from build123d import *

# Parameters (mm, degrees)
CROQUIS1_W              = 44
CROQUIS1_H              = 31
CROQUIS1_R              = 1
CROQUIS1_R_2            = 2.1
SALIENTE_EXTRUIR1_DEPTH = 6
CROQUIS2_W              = 31
CROQUIS2_H              = 6
SALIENTE_EXTRUIR2_DEPTH = 16.5
CROQUIS3_R              = 1.1
CROQUIS3_W              = 20.5
CROQUIS3_H              = 41
SALIENTE_EXTRUIR3_DEPTH = 6
CROQUIS4_R              = 2.1
CROQUIS4_R_2            = 1
SALIENTE_EXTRUIR4_DEPTH = 2
CROQUIS5_R              = 2.1
CORTAR_EXTRUIR1_DEPTH   = 3.5
REDONDEO1_R             = 15.5
CHAFL_N1_SIZE           = 2
CHAFL_N2_SIZE           = 2
CHAFL_N3_SIZE           = 4
CHAFL_N4_SIZE           = 4
CHAFL_N5_SIZE           = 7.5


with BuildPart() as part:
    # Croquis1 → Saliente-Extruir1 (new body)
    with BuildSketch(Plane(origin=(0, 0, 0), x_dir=(1, 0, 0), z_dir=(0, 1, 0))):
        Rectangle(CROQUIS1_W, CROQUIS1_H)
        with Locations(Location((13, 0, 0), (0, 0, 270))):
            Circle(CROQUIS1_R, mode=Mode.SUBTRACT)
        with Locations(Location((0, 0, 0), (0, 0, 270))):
            Circle(CROQUIS1_R_2, mode=Mode.SUBTRACT)
        with Locations(Location((7, 0, 0), (0, 0, 270))):
            Circle(CROQUIS1_R, mode=Mode.SUBTRACT)
        with Locations(Location((-7, 0, 0), (0, 0, 270))):
            Circle(CROQUIS1_R, mode=Mode.SUBTRACT)
        with Locations(Location((-10, 0, 0), (0, 0, 270))):
            Circle(CROQUIS1_R, mode=Mode.SUBTRACT)
        with Locations(Location((-13, 0, 0), (0, 0, 270))):
            Circle(CROQUIS1_R, mode=Mode.SUBTRACT)
        with Locations(Location((-16, 0, 0), (0, 0, 270))):
            Circle(CROQUIS1_R, mode=Mode.SUBTRACT)
        with Locations(Location((10, 0, 0), (0, 0, 270))):
            Circle(CROQUIS1_R, mode=Mode.SUBTRACT)
        with Locations(Location((16, 0, 0), (0, 0, 270))):
            Circle(CROQUIS1_R, mode=Mode.SUBTRACT)
    extrude(amount=SALIENTE_EXTRUIR1_DEPTH)

    # Croquis2 → Saliente-Extruir2 (add)
    with BuildSketch(Plane(origin=(22, 0, 0), x_dir=(0, 0, -1), z_dir=(1, 0, 0))):
        with Locations((0, 3)):
            Rectangle(CROQUIS2_W, CROQUIS2_H)
    extrude(amount=SALIENTE_EXTRUIR2_DEPTH)

    # Croquis3 → Saliente-Extruir3 (add)
    with BuildSketch(Plane(origin=(38.5, 0, 0), x_dir=(0, 0, -1), z_dir=(1, 0, 0))):
        Polygon((15.5, 105), (-14.991801075, 105), (-14.991801075, 6), (-15.5, 6), (-15.5, 0), (15.5, 0), align=None)
        with Locations((-4.741801075, 53.5)):
            Circle(CROQUIS3_R, mode=Mode.SUBTRACT)
        with Locations((-4.741801075, 101.5)):
            Circle(CROQUIS3_R, mode=Mode.SUBTRACT)
        with Locations((5.258198925, 53.5)):
            Circle(CROQUIS3_R, mode=Mode.SUBTRACT)
        with Locations((0.258198925, 77.5)):
            Rectangle(CROQUIS3_W, CROQUIS3_H, mode=Mode.SUBTRACT)
        with Locations((5.258198925, 101.5)):
            Circle(CROQUIS3_R, mode=Mode.SUBTRACT)
    extrude(amount=SALIENTE_EXTRUIR3_DEPTH)

    # Croquis4 → Saliente-Extruir4 (add)
    with BuildSketch(Plane.XZ):
        with Locations(Location((0, 0, 0), (0, 0, 270))):
            Circle(CROQUIS4_R)
        with Locations(Location((0, 0, 0), (0, 0, 270))):
            Circle(CROQUIS4_R_2, mode=Mode.SUBTRACT)
    extrude(amount=-SALIENTE_EXTRUIR4_DEPTH)

    # Croquis5 → Cortar-Extruir1 (cut)
    with BuildSketch(Plane(origin=(0, 6, 0), x_dir=(1, 0, 0), z_dir=(0, 1, 0))):
        with Locations((-13, 0)):
            Circle(CROQUIS5_R)
        with Locations((13, 0)):
            Circle(CROQUIS5_R)
    extrude(amount=-CORTAR_EXTRUIR1_DEPTH, mode=Mode.SUBTRACT)

    # Redondeo1
    redondeo1_edges = [part.edges().sort_by_distance(p)[0] for p in [
        (-22, 3, 15.5),
        (-22, 3, -15.5),
    ]]
    fillet(redondeo1_edges, radius=REDONDEO1_R - 0.0001)  # a hair under: the kernel refuses the full size

    # Chaflán1
    chafl_n1_edges = [part.edges().sort_by_distance(p)[0] for p in [
        (18.99995, 0, 15.5),
        (18.99995, 0, -15.5),
        (-17.460184398, 0, -10.960184398),
        (-17.460184398, 0, 10.960184398),
        (44.5, 52.5, -15.5),
        (44.5, 55.5, 14.991801075),
    ]]
    chamfer(chafl_n1_edges, length=CHAFL_N1_SIZE)

    # Chaflán2
    chafl_n2_edges = [part.edges().sort_by_distance(p)[0] for p in [
        (44.5, 4, 15.5),
    ]]
    chamfer(chafl_n2_edges, length=CHAFL_N2_SIZE)

    # Chaflán3
    chafl_n3_edges = [part.edges().sort_by_distance(p)[0] for p in [
        (44.5, 0, 0),
    ]]
    chamfer(chafl_n3_edges, length=CHAFL_N3_SIZE - 0.0001)  # a hair under: the kernel refuses the full size

    # Chaflán4
    chafl_n4_edges = [part.edges().sort_by_distance(p)[0] for p in [
        (38.5, 6, -0.254099463),
    ]]
    chamfer(chafl_n4_edges, length=CHAFL_N4_SIZE)

    # Chaflán5
    chafl_n5_edges = [part.edges().sort_by_distance(p)[0] for p in [
        (40.5, 105, 14.991801075),
        (40.5, 105, -15.5),
    ]]
    chamfer(chafl_n5_edges, length=CHAFL_N5_SIZE)


solid = part.part
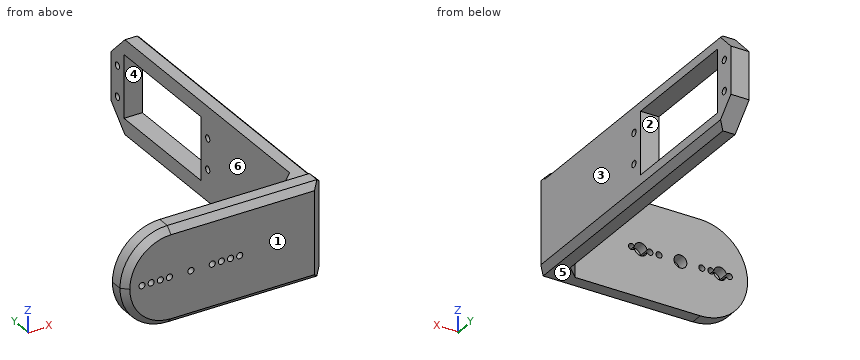
Read the model definition and answer for the solid it produces. Units are mm, in the model's axes. Face numbers are marked on the shaded views. A direction names the side the tool comes from. Round coordinates to 2 decimals unless told otherwise and drop trailing zeros. Order: outer loops, then holes, each group sorted by start corner. A loop starts at its lowest first (then second) coordinate and runs counter-clockwise, first axis right, second up.
1) The mould has two halves that part along Y. Classify the marked faces 1, 2 and 3: released by +Y, released by -Y, zero draft, split by the parting line, or undercut.
2) For the marked faces 4, 5 and 6, determine the directions among +Z, -Z, +X, -X, +Y, -Y from which every point of the face is accessible in a straight line to the end or side of a thin tool.
3) The part is cut by section A-A on y = 84. Write down the section's boundary in (x, z), plus the area to 3 significant figures.
4) The part is cut by section B-B on x = 22.5. Write down the section's boundary in (y, z).
5) Straight lines are drawn through the part: L1, parallel to X at y = 4, z = 0; L2, parallel to Z at x = 10, y = 1.55; L3, parallel to Z at x = 16, y = 4.35. For each, find the intervals that lie inside material, in ascending order.
6) Flat-ended cylindrical pins translate along their axes: pin 1 (1.3 mm diameter, centred on y = 53.5, z = 4.74, fed in from +X); pin 2 (3 mm diameter, centred on x = 7, z = 0, fed in from +Y); pin 3 (15 mm diameter, centred on y = 43.5, z = -6, fed in from -X); pin 4 (6.5 mm diameter, centred on x = 40, y = 83, fed in from +Z). Find the tip coordinate at first contact, or state that the pin passes through.
Resolved:
1. face 1: released by -Y
1. face 2: undercut
1. face 3: zero draft
2. face 4: +X, -X
2. face 5: -Z, +X, -X, +Y, -Y
2. face 6: +Z, -Z, -X, +Y
3. outline: (38.5, -15.5) - (42.5, -15.5) - (44.5, -13.5) - (44.5, -10.51) - (38.5, -10.51) - close; (38.5, 9.99) - (44.5, 9.99) - (44.5, 12.99) - (42.5, 14.99) - (38.5, 14.99) - close
3. area: 56.0 mm2
4. outline: (0, -13.5) - (2, -15.5) - (6, -15.5) - (6, 15.5) - (2, 15.5) - (0, 13.5) - close
5. L1: x = -22 to -17, -9 to -8, -6 to -2.1, 2.1 to 6, 8 to 9, 17 to 44.5
5. L2: z = -15.05 to -1, 1 to 15.05
5. L3: z = -15.5 to -1, 1 to 15.5
6. pin 1: passes through
6. pin 2: stops at y = 6
6. pin 3: stops at x = 38.5
6. pin 4: stops at z = 14.99
